Could you check a few things on this drawing? It's one solid part, dimensions in mm from its lowest x, y, z. A direction names the side the tool comes from. Give positions to 0.01 mm unless a question says otherwise; leave off trailing zeros. Loops run counter-clockwise (first coordinate to the right, second up) from the corner with the lowest first, then second, coordinate; pieces in that order, holes last. Notation, with made-up numbers: (-18, 52) - (-14, 52) arc R22 ccw to (-14, 66) - close; hole circle Ø8 at (49.25, -10). An arc over 180 degrees is marked (long way). Use CSV: the item, a comma, the result in double quotes.
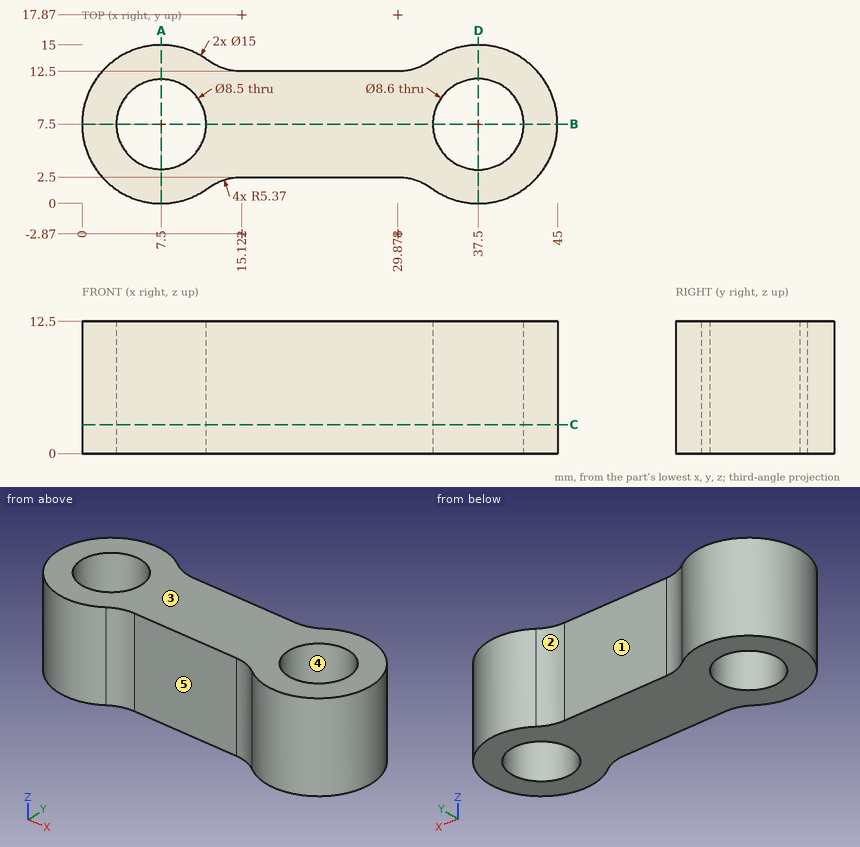
1) I'm going to push flat-ended pins straight in: P1, Ø4, axis at x = 22.5, z = 5, coming from the -Y side; P2, Ø5, axis at x = 37.5, y = 7.5, coming from the +Z side; P3, Ø1.5, axis at y = 9, z = 3, coming from the -X side; P4, Ø1, axis at y = 3, z = 7.5, coming from the -X side (1 decimal). Where does each tip first touch, or does it pass through?
Answer below:
P1,"stops at y = 2.5"
P2,"passes through"
P3,"stops at x = 0.04"
P4,"stops at x = 1.2"
2) Which directions (+Z, -Z, +X, -X, +Y, -Y) give clear straight access to the entire face, cutting with the end or side of a thin tool? Please do the marked faces 4 and 5.
Answer below:
face 4,"+Z, -Z"
face 5,"+Z, -Z, -Y"
3) I need wall thicknesses on line 1 along X through (y, z) = (7.5, 9); line 2 along Y through (x, z) = (37.5, 6.25); line 3 along X through (y, z) = (10.75, 10.5) (1 decimal). Which ranges of each line are inside material? Lowest first, please.
Answer below:
line 1,"x = 0 to 3.25, 11.75 to 33.2, 41.8 to 45"
line 2,"y = 0 to 3.2, 11.8 to 15"
line 3,"x = 0.7 to 4.8, 10.2 to 34.7, 40.3 to 44.3"
4) Suppose I cut it at C-C (z = 2.75). Please give me the cut outline in (x, y), plus the area to 3 significant figures.
Answer below:
outline,"(11.94, 1.46) arc R5.37 cw to (15.12, 2.5) - (29.88, 2.5) arc R5.37 cw to (33.06, 1.46) arc R7.5 ccw (long way) to (33.06, 13.54) arc R5.37 cw to (29.88, 12.5) - (15.12, 12.5) arc R5.37 cw to (11.94, 13.54) arc R7.5 ccw (long way) to start; hole circle Ø8.5 at (7.5, 7.5); hole circle Ø8.6 at (37.5, 7.5)"
area,"402 mm2"
5) We'd pull the mould along X, two halves only. Please class the marked faces 1, 2 and 3: +X half, -X half, draft (parallel to the pull), parting line (faces both ways), or undercut.
Answer below:
face 1,"undercut"
face 2,"undercut"
face 3,"draft"
6) Suppose I cut it at D-D (x = 37.5). Please give me the cut outline in (y, z).
Answer below:
outline,"(0, 0) - (3.2, 0) - (3.2, 12.5) - (0, 12.5) - close; (11.8, 0) - (15, 0) - (15, 12.5) - (11.8, 12.5) - close"
7) Suppose I cut it at B-B (y = 7.5). Please give me the cut outline in (x, z).
Answer below:
outline,"(0, 0) - (3.25, 0) - (3.25, 12.5) - (0, 12.5) - close; (11.75, 0) - (33.2, 0) - (33.2, 12.5) - (11.75, 12.5) - close; (41.8, 0) - (45, 0) - (45, 12.5) - (41.8, 12.5) - close"
8) Suppose I cut it at A-A (x = 7.5). Please give me the cut outline in (y, z).
Answer below:
outline,"(0, 0) - (3.25, 0) - (3.25, 12.5) - (0, 12.5) - close; (11.75, 0) - (15, 0) - (15, 12.5) - (11.75, 12.5) - close"
